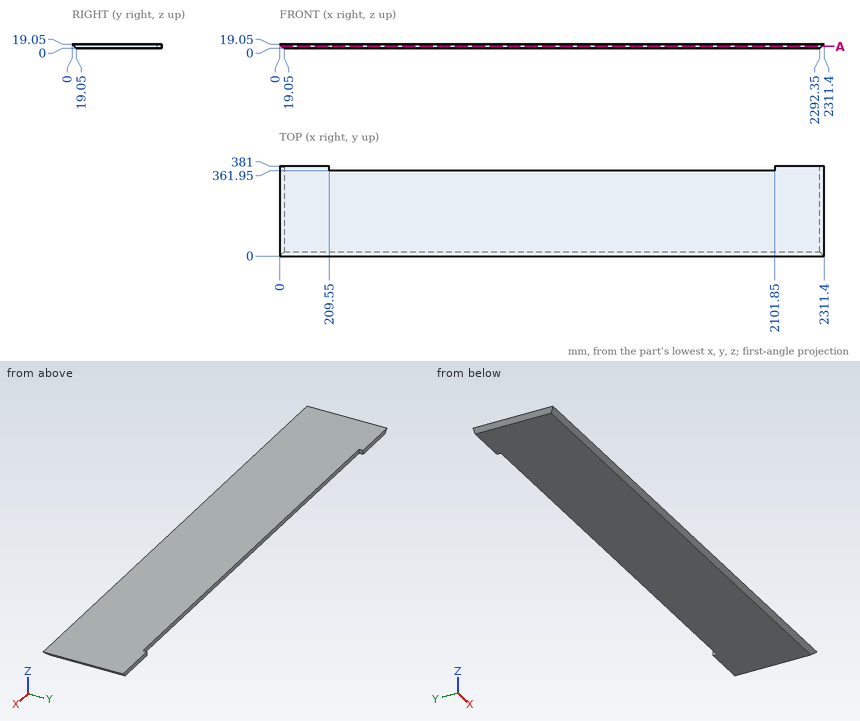
Input: dimensioned drawing with shaded views. Units: mm. Origin: part minimum x, y, z. Coordinates: 2 decimals unless noted, no trailing zeros. Loops run counter-clockwise (first coordinate to the right, second up) from the corner with the lowest first, then second, coordinate; pieces in that order, holes last. Notation, with made-up numbers: M 79.5,-23.5 L 84.5,-23.5 A7 ccw 84.5,-11.5 Z; hole C -36,54.5 d2. An arc over 180 degrees is marked long. Put each result on its own line as item: value.
(1) Material intervals for probe 1 along X at (y, z) = (366, 17); probe 2 along Y at (x, z) = (2098, 8.5); probe 3 along Y at (x, z) = (1746, 5.25), sorted ascending.
Answer sheet:
probe 1: x = 2.05 to 209.55, 2101.85 to 2309.35
probe 2: y = 10.55 to 361.95
probe 3: y = 13.8 to 361.95
(2) First-contact query: pin 1 (5.5 mm diameter, centred on y = 368, z = 13, fed in from +X); pin 2 (5.5 mm diameter, centred on y = 368.5, z = 8.5, fed in from -X); pin 3 (3 mm diameter, centred on y = 148, z = 4, fed in from +X). Flat tips, straight axial feed; report the tip coordinate or a pass-through.
Answer sheet:
pin 1: stops at x = 2308.1
pin 2: stops at x = 7.8
pin 3: stops at x = 2297.85
(3) Cut plane A-A on z = 8.5. Return the cut outline in (x, y).
Answer sheet:
outline: M 10.55,10.55 L 2300.85,10.55 L 2300.85,381 L 2101.85,381 L 2101.85,361.95 L 209.55,361.95 L 209.55,381 L 10.55,381 Z
